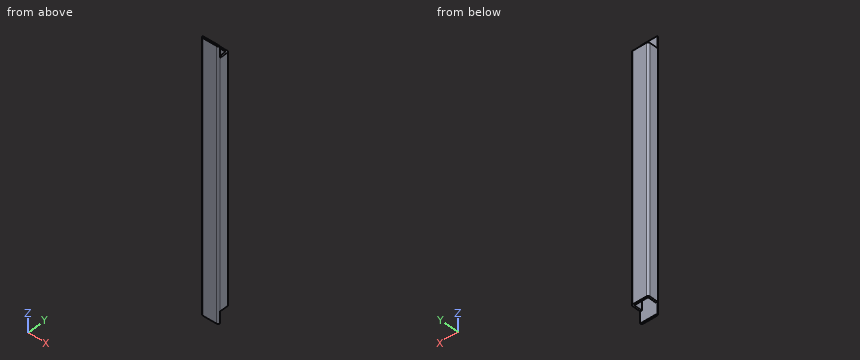
from build123d import *

# Parameters (mm, degrees)
SKETCH1_W           = 24
SKETCH1_H           = 14.34
BOSS_EXTRUDE1_DEPTH = 461
CUT_EXTRUDE1_START  = -20
CUT_EXTRUDE1_DEPTH  = 20
CUT_EXTRUDE2_DEPTH  = 20


with BuildPart() as part:
    # Sketch1 → Boss-Extrude1 (new body)
    with BuildSketch(Plane.XY):
        with BuildLine():
            Line((3, 0), (27, 0))
            ThreePointArc((27, 0), (29.121320344, 0.878679656), (30, 3))
            Line((30, 3), (30, 17.34))
            ThreePointArc((30, 17.34), (29.121320344, 19.461320344), (27, 20.34))
            Line((27, 20.34), (3, 20.34))
            ThreePointArc((3, 20.34), (0.878679656, 19.461320344), (0, 17.34))
            Line((0, 17.34), (0, 3))
            ThreePointArc((0, 3), (0.878679656, 0.878679656), (3, 0))
        make_face()
        with Locations((15, 10.17)):
            Rectangle(SKETCH1_W, SKETCH1_H, mode=Mode.SUBTRACT)
    extrude(amount=BOSS_EXTRUDE1_DEPTH)

    # Sketch2 → Cut-Extrude1 (cut)
    with BuildSketch(Plane.XY.offset(461).offset(CUT_EXTRUDE1_START)):
        with BuildLine():
            Line((3, 3), (0, 3))
            Line((0, 3), (0, 17.34))
            ThreePointArc((0, 17.34), (0.878679656, 19.461320344), (3, 20.34))
            Line((3, 20.34), (27, 20.34))
            ThreePointArc((27, 20.34), (29.121320344, 19.461320344), (30, 17.34))
            Line((30, 17.34), (30, 3))
            Line((30, 3), (27, 3))
            Line((27, 3), (27, 17.34))
            Line((27, 17.34), (3, 17.34))
            Line((3, 17.34), (3, 3))
        make_face()
    extrude(amount=CUT_EXTRUDE1_DEPTH, mode=Mode.SUBTRACT)

    # Sketch3 → Cut-Extrude2 (cut)
    with BuildSketch(Plane(origin=(0, 0, 0), x_dir=(-1, 0, 0), z_dir=(0, 0, -1))):
        with BuildLine():
            Line((-27, 3), (-27, 17.34))
            Line((-27, 17.34), (-3, 17.34))
            Line((-3, 17.34), (-3, 3))
            Line((-3, 3), (0, 3))
            Line((0, 3), (0, 17.34))
            ThreePointArc((0, 17.34), (-0.878679656, 19.461320344), (-3, 20.34))
            Line((-3, 20.34), (-27, 20.34))
            ThreePointArc((-27, 20.34), (-29.121320344, 19.461320344), (-30, 17.34))
            Line((-30, 17.34), (-30, 3))
            Line((-30, 3), (-27, 3))
        make_face()
    extrude(amount=-CUT_EXTRUDE2_DEPTH, mode=Mode.SUBTRACT)


solid = part.part
Read the model definition and answer for the solid it produces. Units are mm, in the model's axes. Give positions to 0.01 mm unless a question says otherwise; leave off trailing zeros. Write each loop counter-clockwise with the first axis right and the second up, starting at its lowest first coordinate (ties: lowest second). Pieces come first, ordered by that corner, then holes. Notation, with made-up numbers: M 8,75 L 29,75 A19 ccw 29,93 Z; hole C 9,81 d7. An arc over 180 degrees is marked long. One line per item, written item: value. Start each with the question number.
(1) Find section C-C (y = 11.25). Determine the outline of the cut face in (x, z), plus the area to 3 significant figures.
(2) Flat-ended cylindrical pins translate along their axes: pin 1 Ø1 at (x, y) = (16.5, 16.5) entering from -Z (3 decimals); pin 2 Ø5 at (x, y) = (12, 17.5) entering from +Z. Find the tip coordinate at first contact, or state that the pin passes through.
(3) Find the intervals of material crossed by line 1 (Y direction, x = 19.25, z = 245); line 2 (X direction, y = 7.5, z = 378.5); line 3 (Z direction, x = 27.25, y = 6.5), in increasing order.
(4) Find section B-B (z = 124). Determine the outline of the cut face in (x, y), plus the area to 3 significant figures.
(5) Find section A-A (x = 7.25). Determine the outline of the cut face in (y, z), plus the area to 3 significant figures.
Results below:
1. outline: M 0,20 L 3,20 L 3,441 L 0,441 Z; M 27,20 L 30,20 L 30,441 L 27,441 Z
1. area: 2,530 mm^2
2. pin 1: passes through
2. pin 2: stops at z = 441
3. line 1: y = 0 to 3, 17.34 to 20.34
3. line 2: x = 0 to 3, 27 to 30
3. line 3: z = 20 to 441
4. outline: M 0,3 A3 ccw 3,0 L 27,0 A3 ccw 30,3 L 30,17.34 A3 ccw 27,20.34 L 3,20.34 A3 ccw 0,17.34 Z; hole M 3,3 L 27,3 L 27,17.34 L 3,17.34 Z
4. area: 258 mm^2
5. outline: M 0,0 L 3,0 L 3,461 L 0,461 Z; M 17.34,20 L 20.34,20 L 20.34,441 L 17.34,441 Z
5. area: 2,650 mm^2
